```python
from build123d import *
from OCP.BRepFilletAPI import BRepFilletAPI_MakeChamfer

# Parameters (mm, degrees)
SKETCH_1_W               = 240
SKETCH_1_H               = 40
EXTRUDE_1_DEPTH          = 5
SKETCH_2_W               = 120
SKETCH_2_H               = 10
EXTRUDE_2_DEPTH          = 50
CHAMFER_1_SIZE           = 20
FILLET_4_R               = 10
CUT_EXTRUDE_1_DEPTH      = 136.369863707
CUT_EXTRUDE_1_DEPTH_BACK = 136.369863707
SKETCH_4_R               = 2.2
CHAMFER_2_SIZE           = 25
CHAMFER_3_SIZE           = 15
CHAMFER_3_SIZE2          = 7.764571353
FILLET_6_R               = 25
FILLET_7_R               = 50
FILLET_8_R               = 50


with BuildPart() as part:
    # 草图1 → 凸台-拉伸1 (new body)
    with BuildSketch(Plane(origin=(0, 0, 0), x_dir=(1, 0, 0), z_dir=(0, 1, 0))):
        Rectangle(SKETCH_1_W, SKETCH_1_H)
    extrude(amount=EXTRUDE_1_DEPTH)

    # 草图2 → 凸台-拉伸2 (add)
    with BuildSketch(Plane(origin=(0, 5, 0), x_dir=(1, 0, 0), z_dir=(0, 1, 0))):
        with Locations((0, 15)):
            Rectangle(SKETCH_2_W, SKETCH_2_H)
    extrude(amount=EXTRUDE_2_DEPTH)

    # 倒角1
    chamfer_1_edges = [part.edges().sort_by_distance(p)[0] for p in [
        (0, 5, -10),
    ]]
    chamfer(chamfer_1_edges, length=CHAMFER_1_SIZE)

    # 圆角4
    fillet_4_edges = [part.edges().sort_by_distance(p)[0] for p in [
        (0, 25, -10),
        (0, 5, 10),
    ]]
    fillet(fillet_4_edges, radius=FILLET_4_R)

    # 草图4 → 切除-拉伸1 (cut, two sides: drawn at the far end of the back side and taken through both)
    with BuildSketch(Plane.XY.offset(-10).offset(-CUT_EXTRUDE_1_DEPTH_BACK)):
        with Locations((-55, 50)):
            Circle(SKETCH_4_R)
        with Locations((55, 50)):
            Circle(SKETCH_4_R)
        with Locations((-55, 25)):
            Circle(SKETCH_4_R)
        with Locations((55, 25)):
            Circle(SKETCH_4_R)
    extrude(amount=CUT_EXTRUDE_1_DEPTH + CUT_EXTRUDE_1_DEPTH_BACK, mode=Mode.SUBTRACT)

    # 倒角2
    chamfer_2_edges = [part.edges().sort_by_distance(p)[0] for p in [
        (120, 2.5, 20),
        (-120, 2.5, 20),
    ]]
    chamfer(chamfer_2_edges, length=CHAMFER_2_SIZE)

    # 倒角3: one chamfer whose edges measure the first distance from different faces: ONE call of the kernel's chamfer builder (chamfer() names one face for all edges)
    chamfer_3_edges_1 = [part.edges().sort_by_distance(p)[0] for p in [
        (120, 2.5, -5),
    ]]
    chamfer_3_side_1 = [part.faces().sort_by_distance(p)[0] for p in [
        (107.5, 2.5, 7.5),
    ]]
    chamfer_3_edges_2 = [part.edges().sort_by_distance(p)[0] for p in [
        (-120, 2.5, -5),
    ]]
    chamfer_3_side_2 = [part.faces().sort_by_distance(p)[0] for p in [
        (-107.5, 2.5, 7.5),
    ]]
    chamfer_3 = BRepFilletAPI_MakeChamfer(part.part.solid().wrapped)
    for e in chamfer_3_edges_1:
        chamfer_3.Add(CHAMFER_3_SIZE, CHAMFER_3_SIZE2, e.wrapped, chamfer_3_side_1[0].wrapped)  # the first distance lies on this face
    for e in chamfer_3_edges_2:
        chamfer_3.Add(CHAMFER_3_SIZE, CHAMFER_3_SIZE2, e.wrapped, chamfer_3_side_2[0].wrapped)  # the first distance lies on this face
    add(Compound.cast(chamfer_3.Shape()), mode=Mode.REPLACE)

    # 圆角6
    fillet_6_edges = [part.edges().sort_by_distance(p)[0] for p in [
        (-120, 2.5, -12.764571353),
        (120, 2.5, -12.764571353),
    ]]
    fillet(fillet_6_edges, radius=FILLET_6_R)

    # 圆角7
    # the kernel refuses this fillet: 50 mm, written as the material it takes off along each edge
    with BuildSketch(Plane(origin=(95, -51.772199057, 20), x_dir=(-1, 0, 0), z_dir=(0, 1, 0))) as fillet_7_piece_1:
        with BuildLine():
            CenterArc((20.708879623, -50), FILLET_7_R, 90, 44.591350674)
            Line((-14.393398282, -14.393398282), (-15.09544384, -13.681266248))
            Line((-15.09544384, -13.681266248), (-0.707106781, 0.707106781))
            Line((-0.707106781, 0.707106781), (0, 1))
            Line((0, 1), (20.708879623, 1))
            Line((20.708879623, 1), (20.708879623, 0))
        make_face()
    extrude(amount=108.544398113, mode=Mode.SUBTRACT)
    with BuildSketch(Plane(origin=(-95, -51.772199057, 20), x_dir=(-0.7071067811865476, 0, -0.7071067811865476), z_dir=(0, 1, 0))) as fillet_7_piece_2:
        with BuildLine():
            CenterArc((20.711949847, -49.998728271), FILLET_7_R, 90.408649326, 44.591350674)
            Line((-14.643389212, -14.643389212), (-15.350495993, -13.936282431))
            Line((-15.350495993, -13.936282431), (-0.707106781, 0.707106781))
            Line((-0.707106781, 0.707106781), (0, 1))
            Line((0, 1), (20.348206844, 0.999974565))
            Line((20.348206844, 0.999974565), (20.355339059, 0))
        make_face()
    extrude(amount=108.544398113, mode=Mode.SUBTRACT)

    # 圆角8
    # the kernel refuses this fillet: 50 mm, written as the material it takes off along each edge
    with BuildSketch(Plane(origin=(109.393398282, -99.666312896, 5.606601718), x_dir=(0.49999999999999956, 0, -0.8660254037844389), z_dir=(0, 1, 0))) as fillet_8_piece_1:
        with BuildLine():
            CenterArc((12.247448714, 50), FILLET_8_R, 210, 60)
            Line((-31.053821475, 25), (-35.383948494, 22.5))
            ThreePointArc((-35.383948494, 22.5), (-34.346314531, 20.702765255), (-1.328508268, -4.820276526))
            Line((-1.328508268, -4.820276526), (0, -5))
            Line((0, -5), (12.247448714, -5))
            Line((12.247448714, -5), (12.247448714, 0))
        make_face()
    extrude(amount=204.332625793, mode=Mode.SUBTRACT)
    with BuildSketch(Plane(origin=(-109.393398282, -99.666312896, 5.606601718), x_dir=(0.9325504463801257, 0, 0.3610396999724933), z_dir=(0, 1, 0))) as fillet_8_piece_2:
        with BuildLine():
            CenterArc((21.81454016, 46.627522319), FILLET_8_R, 231.16406129, 60)
            Line((-9.540086185, 7.680283562), (-12.675548819, 3.785559686))
            Line((-12.675548819, 3.785559686), (-3.135462634, -3.894723876))
            Line((-3.135462634, -3.894723876), (-1.987924813, -4.587826821))
            ThreePointArc((-1.987924813, -4.587826821), (39.736431626, -5.412006342), (41.671723658, -4.662752232))
            Line((41.671723658, -4.662752232), (39.866525159, 0))
        make_face()
    extrude(amount=204.332625793, mode=Mode.SUBTRACT)


solid = part.part
```
Read the model definition and answer for the solid it produces. Units are mm, in the model's axes. A direction names the side the tool comes from. Coordinates: 2 decimals unless noted, no trailing zeros. Write each loop counter-clockwise with the first axis right and the second up, starting at its lowest first coordinate (ties: lowest second). Pieces come first, ordered by that corner, then holes. Notation, with made-up numbers: (70, 69.5) -> (109, 69.5) arc R28 ccw to (109, 102.5) -> close; hole circle Ø11 at (41, 22.25). An arc over 180 degrees is marked (long way). Return JSON: item names as keys, results as strings.
1. A tool of negligible diameter and unlimited length cuts with its end or side. For faces 5 (the face through (-60, 24, -10)), 6 (the face through (-55.477, 47.852, -15.07)), 7 (the face through (-2, 5, 17)), from which of +Z, -Z, +X, -X, +Y, -Y can it reach the whole face along a straight path? Write none if from no direction.
Found:
{"face 5": "+Z, -Z, -X, +Y", "face 6": "+Z, -Z", "face 7": "+Z, +Y"}
2. A cutting plane is placed at C-C (x = -55). Determine the outline of the cut face in (y, z).
Found:
{"outline": "(0, -20) -> (22.8, -20) -> (22.8, -7.73) arc R10 cw to (22.07, -7.07) -> (7.93, 7.07) arc R10 cw to (5, 14.14) -> (5, 20) -> (0, 20) -> close; (27.2, -20) -> (47.8, -20) -> (47.8, -10) -> (29.14, -10) arc R10 cw to (27.2, -9.81) -> close; (52.2, -20) -> (55, -20) -> (55, -10) -> (52.2, -10) -> close"}
3. Determine the mould class of faces 1 (the face through (-55.477, 22.852, -13.944)), 2 (the face through (-2, 0, 0)), 3 (the face through (-1, 55, -15)), 4 (the face through (-1, 42, -10)) for opening direction Y: pulls with the +Y half, pulls with the -Y half, needs draft (parallel to the pull), parting line crosses it, or undercut.
Found:
{"face 1": "undercut", "face 2": "pulls with the -Y half", "face 3": "pulls with the +Y half", "face 4": "needs draft"}
4. Find the intervals of material crossed by line 1 along Y through (x, z) = (55, -17.5); line 2 along X through (y, z) = (50, -15.75); line 3 along X through (y, z) = (9.5, 3), in increasing order. Write a range as from..to.
Found:
{"line 1": "0..22.8, 27.2..47.8, 52.2..55", "line 2": "-60..-57.2, -52.8..52.8, 57.2..60", "line 3": "-60..60"}
5. A cutting plane is placed at D-D (y = 25). Determine the outline of the cut face in (x, z).
Found:
{"outline": "(-60, -20) -> (-57.2, -20) -> (-57.2, -9.1) -> (-60, -9.1) -> close; (-52.8, -20) -> (52.8, -20) -> (52.8, -9.1) -> (-52.8, -9.1) -> close; (57.2, -20) -> (60, -20) -> (60, -9.1) -> (57.2, -9.1) -> close"}
6. A cutting plane is placed at B-B (x = -14). Determine the outline of the cut face in (y, z).
Found:
{"outline": "(0, -20) -> (55, -20) -> (55, -10) -> (29.14, -10) arc R10 cw to (22.07, -7.07) -> (7.93, 7.07) arc R10 cw to (5, 14.14) -> (5, 20) -> (0, 20) -> close"}
7. Each of these flat-tipped pins is pushed along its axis until it touches: P1, Ø1, axis at y = 10.5, z = -13, coming from the -X side; P2, Ø3.5, axis at x = -55, y = 25, coming from the +Z side; P3, Ø6, axis at x = -69.5, z = -3, coming from the +Y side; P4, Ø17, axis at y = 33, z = -7, coming from the +X side. Where does it stop, or does it pass through?
Found:
{"P1": "x = -60", "P2": "through", "P3": "y = 5", "P4": "x = 60"}
8. A cutting plane is placed at A-A (y = 50). Determine the outline of the cut face in (x, z).
Found:
{"outline": "(-60, -20) -> (-57.2, -20) -> (-57.2, -10) -> (-60, -10) -> close; (-52.8, -20) -> (52.8, -20) -> (52.8, -10) -> (-52.8, -10) -> close; (57.2, -20) -> (60, -20) -> (60, -10) -> (57.2, -10) -> close"}
